Autodesk Fusion 360 part; units mm, degrees
sketch "Sketch1" plane through (0, 0, 0) normal (0, 1, 0) x (1, 0, 0)
  line L0 (0, 0) -> (25, 0)
  line L1 (25, 0) -> (25, 22.3)
  line L2 (25, 22.3) -> (0, 22.3)
  line L3 (0, 22.3) -> (0, 0)
  dimension "d1" = 25
  dimension "d2" = 22.3
extrude "Extrude1" add sketch "Sketch1" along normal blind 1.5
fillet "Fillet1" radius 2 4 edges at (25, 0.75, 0) (25, 0.75, -22.3) (0, 0.75, -22.3) (0, 0.75, 0)
sketch "Sketch2" plane through (0, 1.5, 0) normal (0, 1, 0) x (-1, 0, 0)
  arc A0 (0, -2) -> (-2, 0) centre (-2, -2) ccw
  line L0 (-2, 0) -> (-23, 0)
  arc A1 (-23, 0) -> (-25, -2) centre (-23, -2) ccw
  line L1 (-25, -2) -> (-25, -20.3)
  arc A2 (-25, -20.3) -> (-23, -22.3) centre (-23, -20.3) ccw
  line L2 (-23, -22.3) -> (-2, -22.3)
  arc A3 (-2, -22.3) -> (0, -20.3) centre (-2, -20.3) ccw
  line L3 (0, -20.3) -> (0, -2)
  line L4 (0, 0) -> (-2.25, 0)
  line L5 (-2.25, 0) -> (-2.2498, -2.55)
  circle A4 centre (-2.2498, -2.55) radius 1.25
  line L6 (-2.2498, -2.55) -> (-2.2499, -1.275)
  line L7 (-2.2498, -2.55) -> (-2.2498, -19.8)
  circle A5 centre (-2.2498, -19.8) radius 1.25
  line L8 (0, 0) -> (-6.5, 0)
  line L9 (-6.5, 0) -> (-6.5, -0.4982)
  circle A6 centre (-6.44, -2.9975) radius 0.45
  line L10 (-6.44, -2.9975) -> (-9.04, -2.9948)
  circle A7 centre (-9.04, -2.9948) radius 0.45
  line L11 (-9.04, -2.9948) -> (-11.64, -2.9944)
  circle A8 centre (-11.64, -2.9944) radius 0.45
  line L12 (0, 0) -> (-10.75, 0)
  line L13 (-10.75, 0) -> (-10.75, -19)
  circle A9 centre (-10.75, -19) radius 0.6
  line L14 (-9.2, -15.4) -> (-15.7, -15.4)
  line L15 (-15.7, -15.4) -> (-15.7, -12.1)
  line L16 (-15.7, -12.1) -> (-9.2, -12.1)
  line L17 (-9.2, -12.1) -> (-9.2, -15.4)
  line L18 (-3, -9.5) -> (-4.5, -9.5)
  line L19 (-4.5, -9.5) -> (-4.5, -7.5)
  line L20 (-4.5, -7.5) -> (-3, -7.5)
  line L21 (-3, -7.5) -> (-3, -9.5)
  line L22 (-5.5, -9.5) -> (-7, -9.5)
  line L23 (-7, -9.5) -> (-7, -7.5)
  line L24 (-7, -7.5) -> (-5.5, -7.5)
  line L25 (-5.5, -7.5) -> (-5.5, -9.5)
  line L26 (-8, -9.5) -> (-9.5, -9.5)
  line L27 (-9.5, -9.5) -> (-9.5, -7.5)
  line L28 (-9.5, -7.5) -> (-8, -7.5)
  line L29 (-8, -7.5) -> (-8, -9.5)
  line L30 (-14, -7.5) -> (-10.9513, -7.5)
  line L31 (-10.9513, -7.5) -> (-10.9513, -9.2569)
  line L32 (-10.9513, -9.2569) -> (-14, -9.2569)
  line L33 (-14, -9.2569) -> (-14, -7.5)
  line L34 (-17, -10) -> (-19, -10)
  line L35 (-19, -10) -> (-19, -8.5)
  line L36 (-19, -8.5) -> (-17, -8.5)
  line L37 (-17, -8.5) -> (-17, -10)
  line L38 (-17, -7.5) -> (-19, -7.5)
  line L39 (-19, -7.5) -> (-19, -6)
  line L40 (-19, -6) -> (-17, -6)
  line L41 (-17, -6) -> (-17, -7.5)
  line L42 (-11.64, -2.9944) -> (-14.24, -2.9944)
  line L43 (-14.24, -2.9944) -> (-16.84, -2.9944)
  line L44 (-16.84, -2.9944) -> (-19.44, -2.9944)
  circle A10 centre (-14.24, -2.9944) radius 0.45
  circle A11 centre (-16.84, -2.9944) radius 0.45
  circle A12 centre (-19.44, -2.9944) radius 0.45
  dimension "d6" = 2.25
  dimension "d7" = 2.55
  dimension "d8" = 2.5
  dimension "d9" = 17.25
  dimension "d10" = 2.5
  dimension "d11" = 6.5
  dimension "d12" = 2.5
  dimension "d13" = 0.9
  dimension "d14" = 6.5
  dimension "d15" = 2.6
  dimension "d16" = 0.9
  dimension "d17" = 2.6
  dimension "d18" = 0.9
  dimension "d22" = 10.75
  dimension "d23" = 19
  dimension "d24" = 1.2
  dimension "d28" = 2.6
  dimension "d29" = 2.6
  dimension "d30" = 2.6
  dimension "d31" = 0.9
  dimension "d32" = 0.9
  dimension "d33" = 0.9
extrude "Extrude2" cut sketch "Sketch2" against normal blind 5 contours A5 | L5 A4 L6 L7 | L5 A4 L6 L7 | A9
ref_plane "WorkPlane1" through (12.5, 0.75, -11.15) normal (-1, 0, 0) x (0, 0, 1)
mirror "Mirror1" about plane through (12.5, 0.75, -11.15) normal (-1, 0, 0) of "Extrude2"
extrude "Extrude3" add sketch "Sketch2" along normal blind 1 contours L13 L14 L16 L17 | L13 L14 L15 L16 | L18 L19 L20 L21 | L22 L23 L24 L25 | L26 L27 L28 L29 | L30 L31 L32 L33 | L34 L35 L36 L37 | L38 L39 L40 L41
fillet "Fillet2" radius 0.6 12 edges at (9.2, 1.5, -13.75) (15.7, 1.5, -13.75) (8.75, 1.5, -7.5) (8.75, 1.5, -9.5) (6.25, 1.5, -7.5) (6.25, 1.5, -9.5) (3.75, 1.5, -9.5) (3.75, 1.5, -7.5) (19, 1.5, -9.25) (17, 1.5, -9.25) (17, 1.5, -6.75) (19, 1.5, -6.75)
extrude "Extrude4" cut sketch "Sketch2" against normal blind 4 contours A6 | L10 A7 L11 | L10 A7 L11 | A12 | L43 L44 A11 | L43 L44 A11 | L42 L43 A10 | L42 L43 A10 | L11 A8 L42 | L11 A8 L42
The model under review builds one solid part; all positions refer to its coordinate system, in mm. A direction names the side the tool comes from. Give positions to 0.01 mm unless a question says otherwise; leave off trailing zeros. Loops run counter-clockwise (first coordinate to the right, second up) from the corner with the lowest first, then second, coordinate; pieces in that order, holes last. Notation, with made-up numbers: (51, 81) - (79, 81) arc R29 cw to (79, 115) - close; hole circle Ø6 at (19.5, -11.75). An arc over 180 degrees is marked (long way). Answer as a JSON object with one key per item and string values.
Q1. Add section B-B on z = -8. State the section outline as (x, y) points.
Worked out:
{"outline": "(0, 0) - (25, 0) - (25, 1.5) - (14, 1.5) - (14, 2.5) - (10.95, 2.5) - (10.95, 1.5) - (9.5, 1.5) - (9.5, 2.5) - (8, 2.5) - (8, 1.5) - (7, 1.5) - (7, 2.5) - (5.5, 2.5) - (5.5, 1.5) - (4.5, 1.5) - (4.5, 2.5) - (3, 2.5) - (3, 1.5) - (0, 1.5) - close"}
Q2. Add section D-D on z = -19. State the section outline as (x, y) points.
Worked out:
{"outline": "(0, 0) - (1.29, 0) - (1.29, 1.5) - (0, 1.5) - close; (3.21, 0) - (10.15, 0) - (10.15, 1.5) - (3.21, 1.5) - close; (11.35, 0) - (13.65, 0) - (13.65, 1.5) - (11.35, 1.5) - close; (14.85, 0) - (21.79, 0) - (21.79, 1.5) - (14.85, 1.5) - close; (23.71, 0) - (25, 0) - (25, 1.5) - (23.71, 1.5) - close"}
Q3. For faces 4 (the flat face through (12, 2, -9.257)), 5 (the cylindrical face through (19.89, 0.76, -2.97)), 6 (the flat face through (9.5, 2, -9)), 7 (the flat face through (13, 2, -12.1)), 8 (the flat face through (18, 2, -6)), list the 3-axis set-ups (+Z, -Z, +X, -X, +Y, -Y) from which the entire face can be reached by the end or side of a thin tool; tool diameter is ignored.
Worked out:
{"face 4": "+Y", "face 5": "+Y, -Y", "face 6": "+Z, +Y", "face 7": "+X, -X, +Y", "face 8": "+Z, +X, -X, +Y"}
Q4. Insertion check: pin 1 (0.5 mm diameter, centred on x = 18, y = 2, fed in from -Z); pin 2 (0.8 mm diameter, centred on x = 18, y = 2, fed in from +Z); pin 3 (0.5 mm diameter, centred on x = 11, y = 2, fed in from -Z). Each pin has a flat end and moves straight along its axis. Give the tip position at first contact, or say it passes through.
Worked out:
{"pin 1": "stops at z = -10", "pin 2": "stops at z = -6", "pin 3": "stops at z = -15.4"}
Q5. Add section C-C on y = 0.75. Count the separate pieces of the cut face and the enclosed holes in it, plus the area to 3 significant figures.
Worked out:
{"separate pieces": "1", "enclosed holes": "12", "area": "528 mm^2"}
Q6. To check wall thickness, follow line 1 along Z through (x, y) = (10.75, 1.2); line 2 along X through (y, z) = (0.6, -19.5); line 3 along Z through (x, y) = (16.84, 0.6). State the ranges of each line that lie inside material, in increasing order.
Worked out:
{"line 1": "z = -22.3 to -19.6, -18.4 to 0", "line 2": "x = 0 to 1.04, 3.46 to 10.42, 11.08 to 13.92, 14.58 to 21.54, 23.96 to 25", "line 3": "z = -22.3 to -3.44, -2.54 to 0"}
Q7. Mouldability with a two-part tool opening along X and no side actions: class faces 1 (the cylindrical face through (24.43, 0.76, -21.7)), 2 (the flat face through (18, 2.5, -7)), 3 (the cylindrical face through (1.578, 0.76, -18.746)) as +X half, -X half, draft (parallel to the pull), parting line (faces both ways), or undercut.
Worked out:
{"face 1": "+X half", "face 2": "draft", "face 3": "undercut"}
Q8. Add section A-A on x = 6.44. State the section outline as (y, z) points.
Worked out:
{"outline": "(0, -22.3) - (1.5, -22.3) - (1.5, -10.1) arc R0.6 cw to (2.1, -9.5) - (2.5, -9.5) - (2.5, -7.5) - (2.1, -7.5) arc R0.6 cw to (1.5, -6.9) - (1.5, -3.45) - (0, -3.45) - close; (0, -2.55) - (1.5, -2.55) - (1.5, 0) - (0, 0) - close"}
